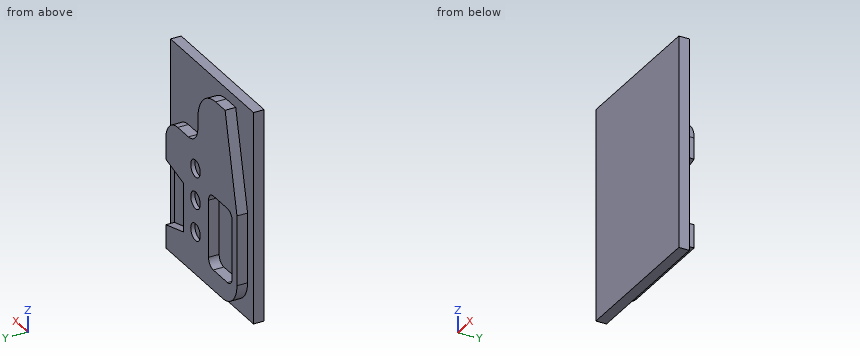
Autodesk Inventor part; units mm, degrees
ref_plane "YZ Plane" through (0, 0, 0) normal (1, 0, 0) x (0, 1, 0)
ref_plane "XZ Plane" through (0, 0, 0) normal (0, 1, 0) x (-1, 0, 0)
ref_plane "XY Plane" through (0, 0, 0) normal (0, 0, 1) x (1, 0, 0)
sketch "Sketch1" plane through (0, 0, 0) normal (0, 1, 0) x (-1, 0, 0)
  line L0 (35, 50) -> (-35, 50)
  line L1 (-35, 50) -> (-35, -50)
  line L2 (-35, -50) -> (35, -50)
  line L3 (35, -50) -> (35, 50)
  line L4 (35, 50) -> (-35, -50) construction
  line L5 (-35, 50) -> (35, -50) construction
  point P0 (0, 0)
  dimension "d0" = 70
  dimension "d1" = 100
extrude "Extrusion1" add sketch "Sketch1" along normal blind 5
sketch "Sketch2" plane through (0, 5, 0) normal (0, 1, 0) x (1, 0, 0)
  line L0 (-20, -45) -> (-12, -45)
  line L1 (30, -7) -> (30, 45)
  line L2 (30, 45) -> (-18, 45)
  line L3 (-30, 33) -> (-30, 0)
  line L4 (-30, -45) -> (30, 45) construction
  line L5 (30, -45) -> (-30, 45) construction
  line L6 (-20, -45) -> (-30, 0)
  line L7 (-35, -50) -> (35, -50)
  line L8 (35, -50) -> (35, 50)
  line L9 (3, -25) -> (3, -30)
  line L10 (20, -17) -> (11, -17)
  arc A0 (11, -17) -> (3, -25) centre (11, -25) ccw
  arc A1 (20, -17) -> (30, -7) centre (20, -7) ccw
  arc A2 (-18, 45) -> (-30, 33) centre (-18, 33) ccw
  line L11 (-22, 0.5) -> (-10, 0.5)
  line L12 (-6, 4.5) -> (-6, 31.5)
  line L13 (-10, 35.5) -> (-22, 35.5)
  line L14 (-26, 31.5) -> (-26, 4.5)
  line L15 (-26, 0.5) -> (-6, 35.5) construction
  line L16 (-6, 0.5) -> (-26, 35.5) construction
  arc A3 (-12, -45) -> (3, -30) centre (-12, -30) ccw
  arc A4 (-26, 4.5) -> (-22, 0.5) centre (-22, 4.5) ccw
  arc A5 (-22, 35.5) -> (-26, 31.5) centre (-22, 31.5) ccw
  arc A6 (-6, 31.5) -> (-10, 35.5) centre (-10, 31.5) ccw
  arc A7 (-10, 0.5) -> (-6, 4.5) centre (-10, 4.5) ccw
  point P0 (0, 0)
  point P1 (3, -45)
  point P2 (-16, 18)
  dimension "d4" = 60
  dimension "d5" = 90
  dimension "d6" = 50
  dimension "d7" = 55
  dimension "d8" = 32
  dimension "d10" = 8
  dimension "d11" = 10
  dimension "d12" = 12
  dimension "d22" = 20
  dimension "d23" = 35
  dimension "d24" = 68
  dimension "d25" = 51
  dimension "d26" = 15
  dimension "d39" = 4
extrude "Extrusion2" add sketch "Sketch2" along normal blind 5
sketch "Sketch3" plane through (0, 10, 0) normal (0, 1, 0) x (1, 0, 0)
  line L0 (15, 7) -> (15, 30)
  line L1 (15, 30) -> (30, 34)
  line L2 (30, -7) -> (30, 45)
  line L3 (15, 7) -> (30, 3)
  line L4 (-35, -50) -> (35, -50)
  line L5 (30, 3) -> (30, 34)
  point P0 (0, 0)
  dimension "d15" = 23
  dimension "d16" = 15
  dimension "d17" = 53
  dimension "d18" = 57
  dimension "d19" = 84
extrude "Extrusion3" cut sketch "Sketch3" against normal blind 4
sketch "Sketch4" plane through (0, 10, 0) normal (0, 1, 0) x (1, 0, 0)
  circle A0 centre (5, -5) radius 4
  line L0 (-35, -50) -> (35, -50)
  line L1 (35, -50) -> (35, 50)
  circle A1 centre (5, 10) radius 4
  circle A2 centre (5, 25) radius 4
  point P0 (0, 0)
  dimension "d27" = 8
  dimension "d28" = 45
  dimension "d29" = 30
  dimension "d32" = 15
extrude "Extrusion4" cut sketch "Sketch4" against normal blind 2
properties part number "A2P4"
Can you work these out from the model? Positions are in its coordinate system, mm. Coordinates: 2 decimals unless noted, no trailing zeros. Order: outer loops, then holes, each group sorted by start corner. A loop starts at its lowest first (then second) coordinate and runs counter-clockwise, first axis right, second up.
1. I'm going to push flat-ended pins straight in: pin 1 (9 mm diameter, centred on x = 6, z = 4.5, fed in from +Y); pin 2 (2 mm diameter, centred on x = -8.5, y = 6.5, fed in from -Z); pin 3 (2.5 mm diameter, centred on y = 8, z = -17.5, fed in from +X); pin 4 (2.5 mm diameter, centred on x = 15.5, y = 8, fed in from +Z). Where does each tip first touch, or does it pass through?
2. If we section it at A-A (x = 16.5): Please give me the cut outline in (y, z), then the cut area to 3 significant figures.
3. I need wall thicknesses on line 1 (X direction, y = 8.55, z = -10); line 2 (X direction, y = 5.25, z = -17); line 3 (Z direction, x = -14, y = 7.5). Which ranges of each line are inside material? Lowest first, please.
4. If we section it at C-C (x = 5): Please give me the cut outline in (y, z).
5. If we section it at B-B (z = -25): Please give me the cut outline in (x, y).
6. If we section it at D-D (z = 5): Please give me the cut outline in (x, y).
Entries:
1. pin 1: stops at y = 10
1. pin 2: stops at z = -45
1. pin 3: stops at x = 15
1. pin 4: stops at z = 17
2. outline: (0, -50) - (5, -50) - (5, -45) - (10, -45) - (10, -30.4) - (6, -30.4) - (6, -6.6) - (10, -6.6) - (10, 17) - (5, 17) - (5, 50) - (0, 50) - close
2. area: 715 mm2
3. line 1: x = -30 to -26, -6 to 1, 9 to 15
3. line 2: x = -30 to -26, -6 to 30
3. line 3: z = -45 to -35.5, -0.5 to 45
4. outline: (0, -50) - (5, -50) - (5, -45) - (10, -45) - (10, -29) - (8, -29) - (8, -21) - (10, -21) - (10, -14) - (8, -14) - (8, -6) - (10, -6) - (10, 1) - (8, 1) - (8, 9) - (10, 9) - (10, 19.71) - (5, 19.71) - (5, 50) - (0, 50) - close
5. outline: (-35, 0) - (35, 0) - (35, 5) - (30, 5) - (30, 6) - (15, 6) - (15, 10) - (9, 10) - (9, 8) - (1, 8) - (1, 10) - (-6, 10) - (-6, 5) - (-26, 5) - (-26, 10) - (-30, 10) - (-30, 5) - (-35, 5) - close
6. outline: (-35, 0) - (35, 0) - (35, 5) - (30, 5) - (30, 10) - (9, 10) - (9, 8) - (1, 8) - (1, 10) - (-28.89, 10) - (-28.89, 5) - (-35, 5) - close
